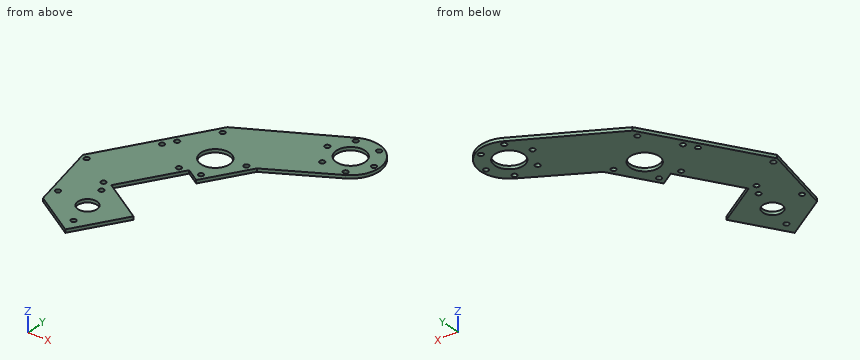
```python
from build123d import *

# Parameters (mm, degrees)
SKETCH1_R              = 14.2875
SKETCH1_R_2            = 9.525
BOSS_EXTRUDE1_DEPTH    = 3.175
F_10_CLEARANCE_HOLE2_D = 4.9784
F_10_CLEARANCE_HOLE3_D = 4.9784


with BuildPart() as part:
    # Sketch1 → Boss-Extrude1 (new body)
    with BuildSketch(Plane.XY.offset(-14.194599474)):
        with BuildLine():
            Line((-11.403602879, 461.040918113), (18.881283072, 509.506866808))
            Line((18.881283072, 509.506866808), (-23.846467356, 536.206128526))
            Line((-23.846467356, 536.206128526), (10.759214603, 591.586796266))
            Line((10.759214603, 591.586796266), (24.22197813, 583.174327946))
            Line((24.22197813, 583.174327946), (51.141876753, 626.255171231))
            Line((51.141876753, 626.255171231), (112.462044501, 660.93728694))
            ThreePointArc((112.462044501, 660.93728694), (123.365099157, 699.702028841), (84.677956887, 710.877306848))
            Line((84.677956887, 710.877306848), (-5.401730059, 661.587538174))
            Line((-5.401730059, 661.587538174), (-69.615486106, 558.824047132))
            Line((-69.615486106, 558.824047132), (-54.307899735, 487.850498283))
            Line((-54.307899735, 487.850498283), (-11.403602879, 461.040918113))
        make_face()
        with Locations((16.14150623, 618.174698631)):
            Circle(SKETCH1_R, mode=Mode.SUBTRACT)
        with Locations((-19.923573493, 500.543719921)):
            Circle(SKETCH1_R_2, mode=Mode.SUBTRACT)
        with Locations((98.394472266, 685.809641802)):
            Circle(SKETCH1_R, mode=Mode.SUBTRACT)
    extrude(amount=BOSS_EXTRUDE1_DEPTH)

    # #10 Clearance Hole2 (through all)
    with Locations(Plane.XY.offset(-11.019599474)):
        with Locations((-25.278710379, 525.37278573), (-14.568436607, 475.714654113), (-3.381611976, 652.837445435), (42.391784014, 624.235053148), (22.201860047, 591.924420685), (-23.571535943, 620.526812972), (-31.474844299, 535.981130963), (-63.785476762, 556.17105493), (-51.664768266, 503.670498499), (2.009121865, 589.566678183), (-30.301510599, 609.756602151)):
            Hole(F_10_CLEARANCE_HOLE2_D / 2)

    # #10 Clearance Hole3 (through all)
    with Locations(Plane.XY.offset(-11.019599474)):
        with Locations((111.013174745, 706.003787092), (122.192466334, 684.978597537), (109.573763855, 664.784452247), (85.775769786, 665.615496512), (74.596478197, 686.640686067), (87.215180677, 706.834831357)):
            Hole(F_10_CLEARANCE_HOLE3_D / 2)


solid = part.part
```
Source: CAD feature listing. Evaluate the final solid. Frame: model axes, mm. Round coordinates to 2 decimals unless told otherwise and drop trailing zeros. Order: outer loops, then holes, each group sorted by start corner. A loop starts at its lowest first (then second) coordinate and runs counter-clockwise, first axis right, second up. Notation, with made-up numbers: (-36, -5.75) -> (17, -5.75) arc R15 cw to (17, 17.25) -> close; hole circle Ø4 at (42.5, 7.5). An arc over 180 degrees is marked (long way). One line per item, written item: value. Start each with the question number.
Q1. Section query A-A (x = 95.5). Return the cut outline in (y, z), plus the area to 3 significant figures.
Q2. Section query D-D (x = -43.5). Return the cut outline in (y, z), plus the area to 3 significant figures.
Q3. Material intervals for probe 1 along Y at (x, z) = (0, -11.8); probe 2 along Y at (x, z) = (-15.5, -11.85); probe 3 along X at (y, z) = (504, -11.4), sorted ascending.
Q4. Section query B-B (z = -13.3). Give the number of separate pieces and of enclosed holes in the cut face, plus the area to 3 significant figures.
Q5. Pin query (flat end, axial travel): pin 1 (8 mm diameter, centred on x = -23.57, y = 620.53, fed in from +Z); pin 2 (1 mm diameter, centred on y = 599, z = -13.5, fed in from +X); pin 3 (1 mm diameter, centred on x = -2.5, z = -12.5, fed in from -Y); pin 4 (1.5 mm diameter, centred on x = 17, z = -13, fed in from +Y). Return the tip coordinate at first contact, or that it passes through.
Q6. Section query C-C (y = 495). Return the cut outline in (x, z), plus the area to 3 significant figures.
Findings below:
1. outline: (651.34, -14.19) -> (671.82, -14.19) -> (671.82, -11.02) -> (651.34, -11.02) -> close; (699.8, -14.19) -> (714.24, -14.19) -> (714.24, -11.02) -> (699.8, -11.02) -> close
1. area: 111 mm²
2. outline: (481.1, -14.19) -> (600.62, -14.19) -> (600.62, -11.02) -> (481.1, -11.02) -> close
2. area: 379 mm²
3. probe 1: 479.29 to 521.31, 574.37 to 588.1, 591.04 to 664.54
3. probe 2: 463.6 to 473.41, 478.02 to 492.11, 508.98 to 530.99, 549.56 to 645.43
3. probe 3: -57.79 to -54.13, -49.2 to -28.8, -11.05 to 15.44
4. separate pieces: 1
4. enclosed holes: 20
4. area: 15,500 mm²
5. pin 1: z = -11.02
5. pin 2: x = 34.42
5. pin 3: y = 474.49
5. pin 4: y = 674.26
6. outline: (-55.85, -14.19) -> (-27.67, -14.19) -> (-27.67, -11.02) -> (-55.85, -11.02) -> close; (-12.18, -14.19) -> (9.82, -14.19) -> (9.82, -11.02) -> (-12.18, -11.02) -> close
6. area: 159 mm²
